Could you check a few things on this model? Use its own coordinates, in mm. A direction names the side the tool comes from. Round coordinates to 2 decimals unless told otherwise and drop trailing zeros. Loops run counter-clockwise (first coordinate to the right, second up) from the corner with the lowest first, then second, coordinate; pieces in that order, holes last. Notation, with made-up numbers: M 10,38 L 53,38 A21 ccw 53,57 Z; hole C -15.75,67.25 d10. An arc over 180 degrees is marked long. One line per item, written item: value. Start each with the question number.
Q1. Imagine slicing it at C-C (x = 16). Please give me the cut outline in (y, z).
Q2. Thinking about a two-plate mould opening in X: for faces 4 (the face through (8.3, 4, 5)), 5 (the face through (2, 10, 6)), 6 (the face through (48, 14, 4)), which applies, released by +X, released by -X, zero draft, split by the parting line, or undercut?
Q3. Imagine slicing it at B-B (y = 10.5). Please give me the cut outline in (x, z), then the cut area to 3 significant figures.
Q4. Imagine slicing it at A-A (z = 4.25). Please give me the cut outline in (x, y).
Q5. Please list where these lines run through material, in increasing order: line 1 along X through (y, z) = (3.75, 4); line 2 along Y through (x, z) = (25.5, 3.5); line 3 along X through (y, z) = (5.5, 6.5).
Q6. I'm going to push flat-ended pins straight in: pin 1 Ø3 at (x, y) = (19.5, 3.5) entering from +Z; pin 2 Ø1.5 at (x, y) = (30, 7) entering from +Z. Where does each tip first touch, or does it pass through?
Q7. Which directions (+Z, -Z, +X, -X, +Y, -Y) give clear straight access to the entire face, cutting with the end or side of a thin tool? Please do faces 1 (the face through (24, 0, 4)), 2 (the face through (21, 24.8, 5)), 3 (the face through (2, 18, 6)).
from build123d import *

# Parameters (mm, degrees)
SKETCH_W        = 48
SKETCH_H        = 28
PAD_DEPTH       = 8
POCKET_DEPTH    = 6
SKETCH002_W     = 4
SKETCH002_H     = 8
POCKET001_DEPTH = 5


with BuildPart() as part:
    # Sketch → Pad (new body)
    with BuildSketch(Plane.XY):
        with Locations((24, 14)):
            Rectangle(SKETCH_W, SKETCH_H)
    extrude(amount=PAD_DEPTH)

    # Sketch001 → Pocket (cut)
    with BuildSketch(Plane.XY.offset(8)):
        with BuildLine():
            Line((3.2, 3.2), (7.7, 3.2))
            Line((7.7, 3.2), (7.7, 4.4))
            ThreePointArc((8.3, 4.4), (8, 4.7), (7.7, 4.4))
            Line((8.3, 4.4), (8.3, 3.2))
            Line((8.3, 3.2), (33.4, 3.2))
            Line((33.4, 3.2), (33.4, 4.4))
            ThreePointArc((34, 4.4), (33.7, 4.7), (33.4, 4.4))
            Line((34, 4.4), (34, 3.2))
            Line((34, 3.2), (44.8, 3.2))
            Line((44.8, 3.2), (44.8, 24.8))
            Line((44.8, 24.8), (34, 24.8))
            Line((34, 24.8), (34, 23.6))
            ThreePointArc((33.4, 23.6), (33.7, 23.3), (34, 23.6))
            Line((33.4, 23.6), (33.4, 24.8))
            Line((33.4, 24.8), (8.3, 24.8))
            Line((8.3, 24.8), (8.3, 23.6))
            ThreePointArc((7.7, 23.6), (8, 23.3), (8.3, 23.6))
            Line((7.7, 23.6), (7.7, 24.8))
            Line((7.7, 24.8), (3.2, 24.8))
            Line((3.2, 24.8), (3.2, 3.2))
        make_face()
    extrude(amount=-POCKET_DEPTH, mode=Mode.SUBTRACT)

    # Sketch002 → Pocket001 (cut)
    with BuildSketch(Plane.XY.offset(8)):
        with Locations((2, 14)):
            Rectangle(SKETCH002_W, SKETCH002_H)
    extrude(amount=-POCKET001_DEPTH, mode=Mode.SUBTRACT)


solid = part.part
Report:
1. outline: M 0,0 L 28,0 L 28,8 L 24.8,8 L 24.8,2 L 3.2,2 L 3.2,8 L 0,8 Z
2. face 4: undercut
2. face 5: zero draft
2. face 6: released by +X
3. outline: M 0,0 L 48,0 L 48,8 L 44.8,8 L 44.8,2 L 3.2,2 L 3.2,3 L 0,3 Z
3. area: 118 mm²
4. outline: M 0,0 L 48,0 L 48,28 L 0,28 L 0,18 L 3.2,18 L 3.2,24.8 L 7.7,24.8 L 7.7,23.6 A0.3 ccw 8.3,23.6 L 8.3,24.8 L 33.4,24.8 L 33.4,23.6 A0.3 ccw 34,23.6 L 34,24.8 L 44.8,24.8 L 44.8,3.2 L 34,3.2 L 34,4.4 A0.3 ccw 33.4,4.4 L 33.4,3.2 L 8.3,3.2 L 8.3,4.4 A0.3 ccw 7.7,4.4 L 7.7,3.2 L 3.2,3.2 L 3.2,10 L 0,10 Z
5. line 1: x = 0 to 3.2, 7.7 to 8.3, 33.4 to 34, 44.8 to 48
5. line 2: y = 0 to 3.2, 24.8 to 28
5. line 3: x = 0 to 3.2, 44.8 to 48
6. pin 1: stops at z = 8
6. pin 2: stops at z = 2
7. face 1: +Z, -Z, +X, -X, -Y
7. face 2: +Z
7. face 3: +Z, -X
